The listing builds one solid part. Answer for the finished solid, in the listing's coordinates (mm). Coordinates: 2 decimals unless noted, no trailing zeros. Order: outer loops, then holes, each group sorted by start corner. A loop starts at its lowest first (then second) coordinate and runs counter-clockwise, first axis right, second up. Notation, with made-up numbers: (40, 33) -> (78, 33) arc R35 ccw to (78, 72) -> close; hole circle Ø5 at (85, 5.25). An arc over 180 degrees is marked (long way). Return JSON: item names as keys, results as strings.
```python
from build123d import *

# Parameters (mm, degrees)
CHAMFER1_SIZE  = 1
CHAMFER1_SIZE2 = 1.732050808
CHAMFER2_SIZE  = 0.5


with BuildPart() as part:
    # Sketch1 → Revolve1 (revolve)
    with BuildSketch(Plane.XY, mode=Mode.PRIVATE) as revolve1_sk:
        Polygon((4.25, 0), (4.25, 9), (8.25, 13), (10.5, 13), (10.5, 8), (7, 8), (7, 0), align=None)
    revolve(revolve1_sk.sketch.rotate(Axis((0, 0, 0), (0, 1, 0)), 90), axis=Axis((0, 0, 0), (0, 1, 0)))

    # Chamfer1
    chamfer1_edges = [part.edges().sort_by_distance(p)[0] for p in [
        (0, 13, 10.5),
    ]]
    chamfer1_side = [part.faces().sort_by_distance(p)[0] for p in [
        (0, 13, 8.546984848),
    ]]
    chamfer(chamfer1_edges, length=CHAMFER1_SIZE, length2=CHAMFER1_SIZE2, reference=chamfer1_side[0])

    # Chamfer2
    chamfer2_edges = [part.edges().sort_by_distance(p)[0] for p in [
        (0, 0, 7),
        (0, 8, 10.5),
    ]]
    chamfer(chamfer2_edges, length=CHAMFER2_SIZE)


solid = part.part
```
Item 1: Determine the mould class of faces 1 (the flat face through (-7, 8, -2)), 2 (the cylindrical face through (6.21, 4.2, -3.23)), 3 (the conical face through (-1.35, 9.25, -4.29)) for opening direction X: pulls with the +X half, pulls with the -X half, needs draft (parallel to the pull), parting line crosses it, or undercut.
Answer list:
{"face 1": "needs draft", "face 2": "parting line crosses it", "face 3": "undercut"}
Item 2: Flat-ended cylindrical pins translate along their axes: pin 1 (2 mm diameter, centred on x = 2, y = 6, fed in from +Z); pin 2 (4 mm diameter, centred on y = 4.5, z = -8, fed in from -X); pin 3 (1 mm diameter, centred on y = 11.5, z = -1.5, fed in from -X). Find the tip coordinate at first contact, or state that the pin passes through.
Answer list:
{"pin 1": "z = 6.93", "pin 2": "x = -3.61", "pin 3": "x = -10.45"}
Item 3: The part is cut by section B-B on x = 0. Determine the outline of the cut face in (y, z).
Answer list:
{"outline": "(0, -6.5) -> (0.5, -7) -> (8, -7) -> (8, -10) -> (8.5, -10.5) -> (11.27, -10.5) -> (13, -9.5) -> (13, -8.25) -> (9, -4.25) -> (0, -4.25) -> close; (0, 4.25) -> (9, 4.25) -> (13, 8.25) -> (13, 9.5) -> (11.27, 10.5) -> (8.5, 10.5) -> (8, 10) -> (8, 7) -> (0.5, 7) -> (0, 6.5) -> close"}
Item 4: The part is cut by section A-A on z = 0. Determine the outline of the cut face in (x, y).
Answer list:
{"outline": "(-10.5, 8.5) -> (-10, 8) -> (-7, 8) -> (-7, 0.5) -> (-6.5, 0) -> (-4.25, 0) -> (-4.25, 9) -> (-8.25, 13) -> (-9.5, 13) -> (-10.5, 11.27) -> close; (4.25, 0) -> (6.5, 0) -> (7, 0.5) -> (7, 8) -> (10, 8) -> (10.5, 8.5) -> (10.5, 11.27) -> (9.5, 13) -> (8.25, 13) -> (4.25, 9) -> close"}
Item 5: The part is cut by section C-C on y = 6.5. Determine the outline of the cut face in (x, z).
Answer list:
{"outline": "circle Ø14 at (0, 0); hole circle Ø8.5 at (0, 0)"}
Item 6: Find the intervals of material crossed by probe 1 along X at (y, z) = (3.25, 0); probe 2 along Y at (x, z) = (8, -3.25); probe 3 along Z at (x, y) = (-1.5, 1), in increasing order.
Answer list:
{"probe 1": "-7 to -4.25, 4.25 to 7", "probe 2": "8 to 13", "probe 3": "-6.84 to -3.98, 3.98 to 6.84"}
